from build123d import *

# Parameters (mm, degrees)
SKETCH1_R           = 1.7
SKETCH1_R_2         = 3.81
BOSS_EXTRUDE1_DEPTH = 3.175


with BuildPart() as part:
    # Sketch1 → Boss-Extrude1 (new body)
    with BuildSketch(Plane.XY):
        with BuildLine():
            Line((-2.081852397, 12.371410211), (-12.371410211, 2.081852397))
            ThreePointArc((-12.371410211, 2.081852397), (-12.773942372, 1.499384559), (-12.944543252, 0.812219176))
            ThreePointArc((-12.944543252, 0.812219176), (-12.97, 0), (-12.944543252, -0.812219176))
            ThreePointArc((-12.944543252, -0.812219176), (-12.773942372, -1.499384559), (-12.371410211, -2.081852397))
            Line((-12.371410211, -2.081852397), (-2.081852397, -12.371410211))
            ThreePointArc((-2.081852397, -12.371410211), (-1.499384559, -12.773942372), (-0.812219176, -12.944543252))
            ThreePointArc((-0.812219176, -12.944543252), (0, -12.97), (0.812219176, -12.944543252))
            ThreePointArc((0.812219176, -12.944543252), (1.499384559, -12.773942372), (2.081852397, -12.371410211))
            Line((2.081852397, -12.371410211), (12.371410211, -2.081852397))
            ThreePointArc((12.371410211, -2.081852397), (12.773942372, -1.499384559), (12.944543252, -0.812219176))
            ThreePointArc((12.944543252, -0.812219176), (12.97, 0), (12.944543252, 0.812219176))
            ThreePointArc((12.944543252, 0.812219176), (12.773942372, 1.499384559), (12.371410211, 2.081852397))
            Line((12.371410211, 2.081852397), (2.081852397, 12.371410211))
            ThreePointArc((2.081852397, 12.371410211), (1.499384559, 12.773942372), (0.812219176, 12.944543252))
            ThreePointArc((0.812219176, 12.944543252), (0, 12.97), (-0.812219176, 12.944543252))
            ThreePointArc((-0.812219176, 12.944543252), (-1.499384559, 12.773942372), (-2.081852397, 12.371410211))
        make_face()
        with Locations((0, -9)):
            Circle(SKETCH1_R, mode=Mode.SUBTRACT)
        with Locations((-9, 0)):
            Circle(SKETCH1_R, mode=Mode.SUBTRACT)
        with Locations((0, 9)):
            Circle(SKETCH1_R, mode=Mode.SUBTRACT)
        with Locations((9, 0)):
            Circle(SKETCH1_R, mode=Mode.SUBTRACT)
        Circle(SKETCH1_R_2, mode=Mode.SUBTRACT)
    extrude(amount=BOSS_EXTRUDE1_DEPTH)


solid = part.part
The model under review builds one solid part; all positions refer to its coordinate system, in mm. Give positions to 0.01 mm unless a question says otherwise; leave off trailing zeros. Write each loop counter-clockwise with the first axis right and the second up, starting at its lowest first coordinate (ties: lowest second). Pieces come first, ordered by that corner, then holes.
1. Draft analysis for pull direction Y (two halves, no side actions). For faces 1 (the cylindrical face through (-10.35, -1.03, 1.57)), 2 (the cylindrical face through (1.51, 12.77, 1.57)), 3 (the flat face through (3, -3, 3.175)), state which applies: +Y half, -Y half, draft (parallel to the pull), parting line (faces both ways), or undercut.
2. Add section D-D, the plane y = -9. Write out the cut boundary in (x, z) (3 decimals), plus the area to 3 significant figures.
3. Add section C-C, the plane z = 2.3. Write out the cut boundary in (x, y), plus the area to 3 significant figures.
4. For P1, Ø4.5, axis at x = 0, y = 9, coming from the +Z side (3 decimals); P2, Ø1.5, axis at x = -3, z = 1, coming from the -Y side; P3, Ø3, axis at x = 0, y = -9, coming from the -Z side, all flat-tipped, find the tip position at first contact; note any pin that passes through.
5. Wall thickness on L1, parallel to Y at x = 0, z = 1.55; L2, parallel to X at y = 1, z = 0.8; L3, parallel to Y at x = 1.5, z = 2.45: over which ranges is each line inside the solid? List them lowest first.
6. Add section A-A, the plane y = 0. Write out the cut boundary in (x, z) (3 decimals).
Worked answers:
1. face 1: undercut
1. face 2: +Y half
1. face 3: draft
2. outline: (-5.453, 0) - (-1.7, 0) - (-1.7, 3.175) - (-5.453, 3.175) - close; (1.7, 0) - (5.453, 0) - (5.453, 3.175) - (1.7, 3.175) - close
2. area: 23.8 mm2
3. outline: (-12.94, -0.81) arc R1.97 ccw to (-12.37, -2.08) - (-2.08, -12.37) arc R1.97 ccw to (-0.81, -12.94) arc R12.97 ccw to (0.81, -12.94) arc R1.97 ccw to (2.08, -12.37) - (12.37, -2.08) arc R1.97 ccw to (12.94, -0.81) arc R12.97 ccw to (12.94, 0.81) arc R1.97 ccw to (12.37, 2.08) - (2.08, 12.37) arc R1.97 ccw to (0.81, 12.94) arc R12.97 ccw to (-0.81, 12.94) arc R1.97 ccw to (-2.08, 12.37) - (-12.37, 2.08) arc R1.97 ccw to (-12.94, 0.81) arc R12.97 ccw to start; hole circle Ø3.4 at (-9, 0); hole circle Ø7.62 at (0, 0); hole circle Ø3.4 at (0, -9); hole circle Ø3.4 at (0, 9); hole circle Ø3.4 at (9, 0)
3. area: 326 mm2
4. P1: stops at z = 3.175
4. P2: stops at y = -12.2
4. P3: passes through
5. L1: y = -12.97 to -10.7, -7.3 to -3.81, 3.81 to 7.3, 10.7 to 12.97
5. L2: x = -12.92 to -10.37, -7.63 to -3.68, 3.68 to 7.63, 10.37 to 12.92
5. L3: y = -12.77 to -9.8, -8.2 to -3.5, 3.5 to 8.2, 9.8 to 12.77
6. outline: (-12.97, 0) - (-10.7, 0) - (-10.7, 3.175) - (-12.97, 3.175) - close; (-7.3, 0) - (-3.81, 0) - (-3.81, 3.175) - (-7.3, 3.175) - close; (3.81, 0) - (7.3, 0) - (7.3, 3.175) - (3.81, 3.175) - close; (10.7, 0) - (12.97, 0) - (12.97, 3.175) - (10.7, 3.175) - close
